Work out the finished part from the listing and answer in its coordinate system (mm). Face numbers are marked on the shaded views. Give positions to 0.01 mm unless a question says otherwise; leave off trailing zeros. Order: outer loops, then holes, each group sorted by start corner. A loop starts at its lowest first (then second) coordinate and runs counter-clockwise, first axis right, second up.
```python
from build123d import *

# Parameters (mm, degrees)
ESQUISSE1_R                  = 48.5
BOSS_EXTRU_1_DEPTH           = 70
ESQUISSE2_R                  = 48.5
ESQUISSE2_R_2                = 47.5
ENL_V_MAT_EXTRU_1_DEPTH      = 10
ESQUISSE3_R                  = 35
ENL_V_MAT_EXTRU_2_DEPTH      = 71
ESQUISSE5_R                  = 45
ESQUISSE5_R_2                = 37
ENL_V_MAT_EXTRU_3_DEPTH      = 68
ESQUISSE6_W                  = 20
ESQUISSE6_H                  = 4.679506057
ENL_V_MAT_EXTRU_5_DEPTH      = 68
BOSS_EXTRU_2_DEPTH           = 10
ESQUISSE9_W                  = 97.082032755
ESQUISSE9_H                  = 83.812700188
ENL_V_MAT_EXTRU_6_DEPTH      = 49.5
ENL_V_MAT_EXTRU_6_DEPTH_BACK = 48.5


with BuildPart() as part:
    # Esquisse1 → Boss.-Extru.1 (new body)
    with BuildSketch(Plane.XY):
        Circle(ESQUISSE1_R)
    extrude(amount=BOSS_EXTRU_1_DEPTH)

    # Esquisse2 → Enlèv. mat.-Extru.1 (cut)
    with BuildSketch(Plane.XY.offset(70)):
        Circle(ESQUISSE2_R)
        Circle(ESQUISSE2_R_2, mode=Mode.SUBTRACT)
    extrude(amount=-ENL_V_MAT_EXTRU_1_DEPTH, mode=Mode.SUBTRACT)

    # Esquisse3 → Enlèv. mat.-Extru.2 (cut, through all)
    with BuildSketch(Plane.XY.offset(70)):
        Circle(ESQUISSE3_R)
    extrude(amount=-ENL_V_MAT_EXTRU_2_DEPTH, mode=Mode.SUBTRACT)

    # Esquisse5 → Enlèv. mat.-Extru.3 (cut)
    with BuildSketch(Plane(origin=(0, 0, 0), x_dir=(-1, 0, 0), z_dir=(0, 0, -1))):
        Circle(ESQUISSE5_R)
        Circle(ESQUISSE5_R_2, mode=Mode.SUBTRACT)
    extrude(amount=-ENL_V_MAT_EXTRU_3_DEPTH, mode=Mode.SUBTRACT)

    # Esquisse6 → Enlèv. mat.-Extru.5 (cut)
    with BuildSketch(Plane(origin=(0, 0, 0), x_dir=(-1, 0, 0), z_dir=(0, 0, -1))):
        with Locations((0, -46.214574966)):
            Rectangle(ESQUISSE6_W, ESQUISSE6_H)
    extrude(amount=-ENL_V_MAT_EXTRU_5_DEPTH, mode=Mode.SUBTRACT)

    # Esquisse8 → Boss.-Extru.2 (add)
    with BuildSketch(Plane(origin=(0, 0, 0), x_dir=(-1, 0, 0), z_dir=(0, 0, -1))):
        with BuildLine():
            ThreePointArc((34.294678888, -34.294678888), (48.5, 0), (34.294678888, 34.294678888))
            Line((34.294678888, 34.294678888), (31.819805153, 31.819805153))
            ThreePointArc((31.819805153, 31.819805153), (45, 0), (31.819805153, -31.819805153))
            Line((31.819805153, -31.819805153), (34.294678888, -34.294678888))
        make_face()
        with BuildLine():
            ThreePointArc((-34.294678888, -34.294678888), (-48.5, 0), (-34.294678888, 34.294678888))
            Line((-34.294678888, 34.294678888), (-31.819805153, 31.819805153))
            ThreePointArc((-31.819805153, 31.819805153), (-45, 0), (-31.819805153, -31.819805153))
            Line((-31.819805153, -31.819805153), (-34.294678888, -34.294678888))
        make_face()
    extrude(amount=BOSS_EXTRU_2_DEPTH)

    # Esquisse9 → Enlèv. mat.-Extru.6 (cut, two sides)
    with BuildSketch(Plane(origin=(0, 0, 0), x_dir=(1, 0, 0), z_dir=(0, 1, 0))) as enl_v_mat_extru_6_sk:
        with Locations((0.041016378, -18.093649906)):
            Rectangle(ESQUISSE9_W, ESQUISSE9_H)
    extrude(amount=ENL_V_MAT_EXTRU_6_DEPTH, mode=Mode.SUBTRACT)
    extrude(enl_v_mat_extru_6_sk.sketch, amount=-ENL_V_MAT_EXTRU_6_DEPTH_BACK, mode=Mode.SUBTRACT)


solid = part.part
```
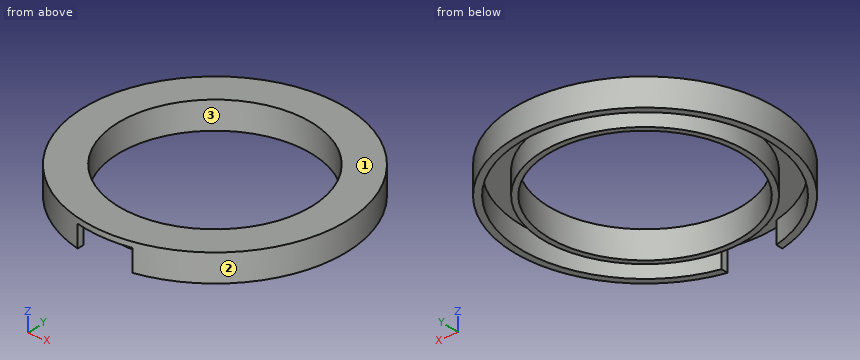
1. The part is cut by section D-D (x = 40). Write down the section's boundary in (y, z), then the cut area to 3 significant figures.
Findings below:
outline: (-25.62, 60) - (-20.62, 60) - (-20.62, 68) - (20.62, 68) - (20.62, 60) - (25.62, 60) - (25.62, 70) - (-25.62, 70) - close
area: 182 mm2
2. The mould has two halves that part along X. Classify the marked faces 1, 2 and 3: pulls with the +X half, pulls with the -X half, needs draft (parallel to the pull), parting line crosses it, or undercut.
Findings below:
face 1: needs draft
face 2: parting line crosses it
face 3: undercut
3. Given P1, Ø4, axis at x = 21, y = -37, coming from the -Z side; P2, Ø6, axis at y = -19.5, z = 61, coming from the +X side; P3, Ø1, axis at x = 15, z = 61.5, coming from the -Y side, each flat-ended and moving along its own axis, determine where each tip first touches the part or whether it passes through.
Findings below:
P1: stops at z = 68
P2: stops at x = 44.54
P3: stops at y = -45.23
4. The part is cut by section C-C (x = 0). Write down the section's boundary in (y, z).
Findings below:
outline: (-47.5, 68) - (-37, 68) - (-37, 60) - (-35, 60) - (-35, 70) - (-47.5, 70) - close; (35, 60) - (37, 60) - (37, 68) - (45, 68) - (45, 60) - (47.5, 60) - (47.5, 70) - (35, 70) - close
5. The part is cut by section B-B (y = -3). Write down the section's boundary in (x, z).
Findings below:
outline: (-47.41, 60) - (-44.9, 60) - (-44.9, 68) - (-36.88, 68) - (-36.88, 60) - (-34.87, 60) - (-34.87, 70) - (-47.41, 70) - close; (34.87, 60) - (36.88, 60) - (36.88, 68) - (44.9, 68) - (44.9, 60) - (47.41, 60) - (47.41, 70) - (34.87, 70) - close
6. The part is cut by section A-A (z = 63.25). Write down the section's boundary in (x, y).
Findings below:
outline: circle Ø74 at (0, 0); (-10, -46.44) - (-10, -43.87) arc R45 cw (long way) to (10, -43.87) - (10, -46.44) arc R47.5 ccw (long way) to start; hole circle Ø70 at (0, 0)
7. Straight lines are drawn through the part: probe 1 along X at (y, z) = (0, 64.75); probe 2 along Y at (x, z) = (0, 65.25); probe 3 along Y at (x, z) = (-20, 65.5). For each, find the intervals that lie inside material, in ascending order.
Findings below:
probe 1: x = -47.5 to -45, -37 to -35, 35 to 37, 45 to 47.5
probe 2: y = -37 to -35, 35 to 37, 45 to 47.5
probe 3: y = -43.08 to -40.31, -31.13 to -28.72, 28.72 to 31.13, 40.31 to 43.08
